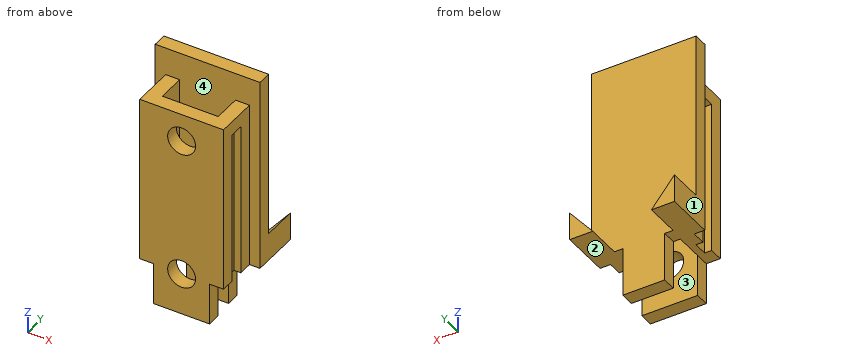
from build123d import *

# Parameters (mm, degrees)
SKETCH1_W            = 7.5
SKETCH1_H            = 10
BOSS_EXTRUDE1_DEPTH  = 1
BOSS_EXTRUDE2_DEPTH  = 2.5
SKETCH10_W           = 7.5
SKETCH10_H           = 1
BOSS_EXTRUDE5_DEPTH  = 2
SKETCH56_W           = 7.5
SKETCH56_H           = 1
BOSS_EXTRUDE17_DEPTH = 2
SKETCH57_W           = 3
SKETCH57_H           = 1
BOSS_EXTRUDE18_DEPTH = 5
SKETCH58_W           = 1.5
SKETCH58_H           = 1
BOSS_EXTRUDE19_DEPTH = 2
SKETCH59_W           = 1.5
SKETCH59_H           = 1
BOSS_EXTRUDE20_DEPTH = 2
SKETCH60_W           = 1
SKETCH60_H           = 1.5
BOSS_EXTRUDE23_DEPTH = 1.5
SKETCH61_W           = 1
SKETCH61_H           = 0.75
CUT_EXTRUDE1_DEPTH   = 0.5
SKETCH62_W           = 6
SKETCH62_H           = 12
BOSS_EXTRUDE25_DEPTH = 3
SKETCH64_W           = 4
SKETCH64_H           = 2
CUT_EXTRUDE2_DEPTH   = 12
SKETCH65_W           = 4
SKETCH65_H           = 1
BOSS_EXTRUDE26_DEPTH = 3
SKETCH66_R           = 1
CUT_EXTRUDE3_DEPTH   = 1
SKETCH68_W           = 6
SKETCH68_H           = 1
SKETCH68_W_2         = 3
SKETCH68_W_3         = 2
CUT_EXTRUDE6_DEPTH   = 0.5
SKETCH67_W           = 6
SKETCH67_H           = 1
SKETCH67_W_2         = 3
SKETCH67_W_3         = 2
CUT_EXTRUDE7_DEPTH   = 0.5
SKETCH69_W           = 7
SKETCH69_H           = 1.5
CUT_EXTRUDE8_DEPTH   = 10


with BuildPart() as part:
    # Sketch1 → Boss-Extrude1 (new body)
    with BuildSketch(Plane(origin=(0, 0, 0), x_dir=(1, 0, 0), z_dir=(0, 1, 0))):
        Rectangle(SKETCH1_W, SKETCH1_H)
    extrude(amount=BOSS_EXTRUDE1_DEPTH)

    # Sketch2 → Boss-Extrude2 (add)
    with BuildSketch(Plane(origin=(0, 1, 0), x_dir=(1, 0, 0), z_dir=(0, 1, 0))):
        Polygon((-3.75, 3), (-2.1, 5), (-3.75, 5), align=None)
        Polygon((3.75, 5), (2.1, 5), (3.75, 3), align=None)
    extrude(amount=BOSS_EXTRUDE2_DEPTH)

    # Sketch10 → Boss-Extrude5 (add)
    with BuildSketch(Plane.XY.offset(5)):
        with Locations((0, 0.5)):
            Rectangle(SKETCH10_W, SKETCH10_H)
    extrude(amount=BOSS_EXTRUDE5_DEPTH)

    # Sketch56 → Boss-Extrude17 (add)
    with BuildSketch(Plane.XY.offset(7)):
        with Locations((0, 0.5)):
            Rectangle(SKETCH56_W, SKETCH56_H)
    extrude(amount=BOSS_EXTRUDE17_DEPTH)

    # Sketch57 → Boss-Extrude18 (add)
    with BuildSketch(Plane(origin=(0, 0, -5), x_dir=(-1, 0, 0), z_dir=(0, 0, -1))):
        with Locations((0, 0.5)):
            Rectangle(SKETCH57_W, SKETCH57_H)
    extrude(amount=BOSS_EXTRUDE18_DEPTH)

    # Sketch58 → Boss-Extrude19 (add)
    with BuildSketch(Plane(origin=(1.5, 0, 0), x_dir=(0, 0, -1), z_dir=(1, 0, 0))):
        with Locations((9.25, 0.5)):
            Rectangle(SKETCH58_W, SKETCH58_H)
    extrude(amount=BOSS_EXTRUDE19_DEPTH)

    # Sketch59 → Boss-Extrude20 (add)
    with BuildSketch(Plane.ZY.offset(1.5)):
        with Locations((-9.25, 0.5)):
            Rectangle(SKETCH59_W, SKETCH59_H)
    extrude(amount=BOSS_EXTRUDE20_DEPTH)

    # Sketch60 → Boss-Extrude23 (add)
    with BuildSketch(Plane(origin=(0, 1, 0), x_dir=(1, 0, 0), z_dir=(0, 1, 0))):
        with Locations((3, 9.25)):
            Rectangle(SKETCH60_W, SKETCH60_H)
        with Locations((-3, 9.25)):
            Rectangle(SKETCH60_W, SKETCH60_H)
    extrude(amount=BOSS_EXTRUDE23_DEPTH)

    # Sketch61 → Cut-Extrude1 (cut)
    with BuildSketch(Plane(origin=(0, 2.5, 0), x_dir=(1, 0, 0), z_dir=(0, 1, 0))):
        with Locations((-3, 9.245443114)):
            Rectangle(SKETCH61_W, SKETCH61_H)
        with Locations((3, 9.245443114)):
            Rectangle(SKETCH61_W, SKETCH61_H)
    extrude(amount=-CUT_EXTRUDE1_DEPTH, mode=Mode.SUBTRACT)

    # Sketch62 → Boss-Extrude25 (add)
    with BuildSketch(Plane(origin=(0, 0, 0), x_dir=(-1, 0, 0), z_dir=(0, -1, 0))):
        with Locations((0, -1)):
            Rectangle(SKETCH62_W, SKETCH62_H)
    extrude(amount=BOSS_EXTRUDE25_DEPTH)

    # Sketch64 → Cut-Extrude2 (cut)
    with BuildSketch(Plane.XY.offset(7)):
        with Locations((0, -1)):
            Rectangle(SKETCH64_W, SKETCH64_H)
    extrude(amount=-CUT_EXTRUDE2_DEPTH, mode=Mode.SUBTRACT)

    # Sketch65 → Boss-Extrude26 (add)
    with BuildSketch(Plane(origin=(0, 0, -5), x_dir=(-1, 0, 0), z_dir=(0, 0, -1))):
        with Locations((0, -2.5)):
            Rectangle(SKETCH65_W, SKETCH65_H)
    extrude(amount=BOSS_EXTRUDE26_DEPTH)

    # Sketch66 → Cut-Extrude3 (cut)
    with BuildSketch(Plane(origin=(0, -3, 0), x_dir=(-1, 0, 0), z_dir=(0, -1, 0))):
        with Locations(Location((0, -5, 0), (0, 0, 90))):  # turned: the seam where the file's is
            Circle(SKETCH66_R)
        with Locations(Location((0, 5, 0), (0, 0, 90))):  # turned: the seam where the file's is
            Circle(SKETCH66_R)
    extrude(amount=-CUT_EXTRUDE3_DEPTH, mode=Mode.SUBTRACT)

    # Sketch68 → Cut-Extrude6 (cut)
    with BuildSketch(Plane(origin=(3, 0, 0), x_dir=(0, 0, -1), z_dir=(1, 0, 0))):
        with Locations((-3, -1.5)):
            Rectangle(SKETCH68_W, SKETCH68_H)
        with Locations((1.5, -1.5)):
            Rectangle(SKETCH68_W_2, SKETCH68_H)
        with Locations((4, -1.5)):
            Rectangle(SKETCH68_W_3, SKETCH68_H)
    extrude(amount=-CUT_EXTRUDE6_DEPTH, mode=Mode.SUBTRACT)

    # Sketch67 → Cut-Extrude7 (cut)
    with BuildSketch(Plane.ZY.offset(3)):
        with Locations((3, -1.5)):
            Rectangle(SKETCH67_W, SKETCH67_H)
        with Locations((-1.5, -1.5)):
            Rectangle(SKETCH67_W_2, SKETCH67_H)
        with Locations((-4, -1.5)):
            Rectangle(SKETCH67_W_3, SKETCH67_H)
    extrude(amount=-CUT_EXTRUDE7_DEPTH, mode=Mode.SUBTRACT)

    # Sketch69 → Cut-Extrude8 (cut)
    with BuildSketch(Plane.XZ):
        with Locations((0, -9.25)):
            Rectangle(SKETCH69_W, SKETCH69_H)
    extrude(amount=-CUT_EXTRUDE8_DEPTH, mode=Mode.SUBTRACT)


solid = part.part
Model file for the job. Use its own axes, mm. Face numbers are marked on the shaded views. Round coordinates to 2 decimals unless told otherwise and drop trailing zeros. Loops run counter-clockwise (first coordinate to the right, second up) from the corner with the lowest first, then second, coordinate; pieces in that order, holes last.
1. Band-saw the part on B-B, the plane z = -2.5. List the corners of the cut face in (x, y), and give its area (3 significant figures).
Check values:
outline: (-3.75, 0) - (-3, 0) - (-3, -1) - (-2.5, -1) - (-2.5, -2) - (-3, -2) - (-3, -3) - (3, -3) - (3, -2) - (2.5, -2) - (2.5, -1) - (3, -1) - (3, 0) - (3.75, 0) - (3.75, 1) - (-3.75, 1) - close; hole (-2, -2) - (2, -2) - (2, 0) - (-2, 0) - close
area: 16.5 mm2
2. Wall check: probe 1 along X at (y, z) = (-2.35, 5); probe 2 along X at (y, z) = (-1.75, 5.5); probe 3 along Y at (x, z) = (-0.75, -2.75). Give the ranges that are in metal, low to high.
Check values:
probe 1: x = -3 to -1, 1 to 3
probe 2: x = -2.5 to -2, 2 to 2.5
probe 3: y = -3 to -2, 0 to 1
3. Mould opens along X. For the marked faces 1, 2, 3 and 4 say: +X half, -X half, draft (parallel to the pull), parting line (faces both ways), or undercut.
Check values:
face 1: -X half
face 2: draft
face 3: undercut
face 4: undercut
4. Band-saw the part on C-C, the plane y = 1.25. List the corners of the cut face in (x, z).
Check values:
outline: (-3.75, -5) - (-2.1, -5) - (-3.75, -3) - close; (2.1, -5) - (3.75, -5) - (3.75, -3) - close
5. Band-saw the part on D-D, the plane y = -1.5. List the corners of the cut face in (x, z), and give its area (3 significant figures).
Check values:
outline: (-3, 6) - (-2.5, 6) - (-2.5, -5) - (-2, -5) - (-2, 7) - (-3, 7) - close; (2, -5) - (2.5, -5) - (2.5, 6) - (3, 6) - (3, 7) - (2, 7) - close
area: 13.0 mm2
6. Band-saw the part on A-A, the plane x = 0. List the corners of the cut face in (y, z).
Check values:
outline: (-3, -8) - (-2, -8) - (-2, -6) - (-3, -6) - close; (-3, -4) - (-2, -4) - (-2, 4) - (-3, 4) - close; (-3, 6) - (-2, 6) - (-2, 7) - (-3, 7) - close; (0, -8.5) - (1, -8.5) - (1, 9) - (0, 9) - close
7. Drop flat-ended pins along their axis: P1, Ø0.8, axis at y = -2.5, z = -7, coming from the +X side; P2, Ø2, axis at y = -1.5, z = 2, coming from the -X side; P3, Ø2, axis at x = 0.5, z = -2.5, coming from the +Y side. Give the stop position or say it passes through.
Check values:
P1: stops at x = 2
P2: stops at x = -3
P3: stops at y = 1
